Geometry: final body of the model. Coordinates: model frame, mm. Face numbers are marked on the shaded views. A direction names the side the tool comes from. Round coordinates to 2 decimals unless told otherwise and drop trailing zeros. Loops run counter-clockwise (first coordinate to the right, second up) from the corner with the lowest first, then second, coordinate; pieces in that order, holes last. Notation, with made-up numbers: M 5,54 L 27,54 A31 ccw 27,91 Z; hole C 36,48.25 d11. An arc over 180 degrees is marked long. Answer as a JSON object with one key per item and string values.
Autodesk Inventor part; units mm, degrees
ref_plane "YZ Plane" through (0, 0, 0) normal (1, 0, 0) x (0, 1, 0)
ref_plane "XZ Plane" through (0, 0, 0) normal (0, 1, 0) x (-1, 0, 0)
ref_plane "XY Plane" through (0, 0, 0) normal (0, 0, 1) x (1, 0, 0)
sketch "Sketch1" plane through (0, 0, 0) normal (0, 1, 0) x (-1, 0, 0)
  line L0 (0, 0) -> (9, 0)
  line L1 (9, 0) -> (9, -6.12)
  line L2 (9, -6.12) -> (0, -6.12)
  line L3 (0, -6.12) -> (0, 0)
  dimension "d0" = 6.12
  dimension "d1" = 9
extrude "Extrusion1" add sketch "Sketch1" along normal blind 5
sketch "Sketch2" plane through (0, 0, 0) normal (1, 0, 0) x (0, 0, -1)
  circle A0 centre (2.6, 2.5) radius 1.925
  circle A1 centre (2.6, 2.5) radius 0.675
  line L0 (6.12, 0) -> (0, 0)
  line L1 (0, 5) -> (6.12, 5)
  line L2 (0, 0) -> (0, 5)
  dimension "d4" = 3.85
  dimension "d5" = 1.35
  dimension "d6" = 5
  dimension "d7" = 2.5
  dimension "d8" = 2.6
extrude "Extrusion2" cut sketch "Sketch2" against normal blind 7
equation "\"d7\" = 0.5 * d6"
properties part number "Barrel Jack small"
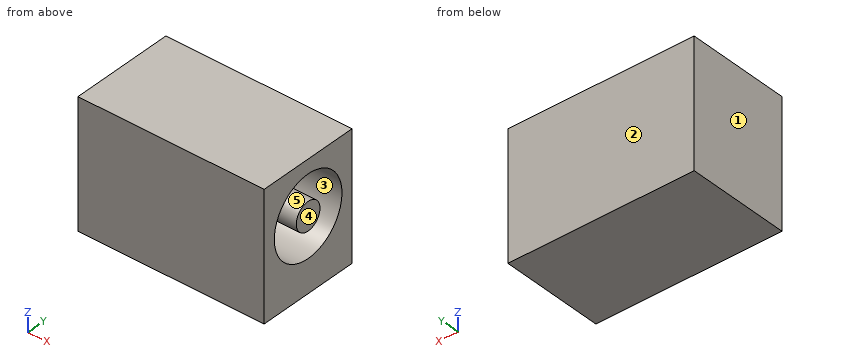
1) Section query A-A (y = 2.5). Return the cut outline in (x, z) (3 decimals), and give its area (3 significant figures).
Results:
{"outline": "M -9,-6.12 L 0,-6.12 L 0,-4.525 L -7,-4.525 L -7,-3.275 L 0,-3.275 L 0,-1.925 L -7,-1.925 L -7,-0.675 L 0,-0.675 L 0,0 L -9,0 Z", "area": "37.6 mm2"}
2) Section query B-B (z = -2.6). Return the cut outline in (x, y) (3 decimals), and give its area (3 significant figures).
Results:
{"outline": "M -9,0 L 0,0 L 0,0.575 L -7,0.575 L -7,1.825 L 0,1.825 L 0,3.175 L -7,3.175 L -7,4.425 L 0,4.425 L 0,5 L -9,5 Z", "area": "27.5 mm2"}
3) Section query D-D (z = -4). Return the cut outline in (x, y).
Results:
{"outline": "M -9,0 L 0,0 L 0,1.18 L -7,1.18 L -7,3.82 L 0,3.82 L 0,5 L -9,5 Z"}
4) Ray query, line 1 (Y direction, x = -3.5, z = -2.6) (3 decimals); line 2 (Y direction, x = -3, z = -2.25); line 3 (X direction, y = 1.7, z = -3.25). Return the intervals inside material, ascending.
Results:
{"line 1": "0 to 0.575, 1.825 to 3.175, 4.425 to 5", "line 2": "0 to 0.61, 1.92 to 3.08, 4.39 to 5", "line 3": "-9 to -7"}
5) Reachability of the marked faces 4 and 5 from +Z, -Z, +X, -X, +Y, -Y: full face, straight path, thin tool, end or side. Return the list, or none.
Results:
{"face 4": "+Z, -Z, +X, +Y, -Y", "face 5": "+X"}
6) Pin query (flat end, axial travel): P1, Ø1.9, axis at y = 3, z = -3, coming from the +X side. Return the tip coordinate at first contact, or that it passes through.
Results:
{"P1": "x = 0"}
7) Pull-direction query (Y, two-part tool) for the marked faces 1, 2 and 3; classes: +Y half, -Y half, draft (parallel to the pull), parting line (faces both ways), or undercut.
Results:
{"face 1": "draft", "face 2": "+Y half", "face 3": "undercut"}
8) Section query C-C (y = 3.85). Return the cut outline in (x, z), and give its area (3 significant figures).
Results:
{"outline": "M -9,-6.12 L 0,-6.12 L 0,-3.97 L -7,-3.97 L -7,-1.23 L 0,-1.23 L 0,0 L -9,0 Z", "area": "35.9 mm2"}
